Autodesk Inventor part; units mm, degrees
ref_plane "YZ Plane" through (0, 0, 0) normal (1, 0, 0) x (0, 1, 0)
ref_plane "XZ Plane" through (0, 0, 0) normal (0, 1, 0) x (-1, 0, 0)
ref_plane "XY Plane" through (0, 0, 0) normal (0, 0, 1) x (1, 0, 0)
sketch "Sketch1" plane through (0, 0, 0) normal (0, 0, 1) x (1, 0, 0)
  line L0 (229.6952, -414.7737) -> (228.902, -414.7737)
  line L1 (204.202, -567.6898) -> (204.202, -542.0358)
  line L2 (204.202, -542.0358) -> (229.856, -542.0358)
  line L3 (204.202, -567.6898) -> (-74.944, -567.6898)
  line L4 (-74.944, -567.6898) -> (-74.944, -265.633)
  line L5 (229.856, -542.0358) -> (229.856, -8.8898)
  line L6 (229.856, -8.8898) -> (188.7123, -8.8898)
  circle A0 centre (20.5783, -308.8638) radius 3.5687
  circle A1 centre (20.574, -385.0638) radius 3.5687
  circle A2 centre (20.574, -461.2638) radius 3.5687
  circle A3 centre (20.574, -537.4638) radius 3.5687
  circle A4 centre (217.156, -529.3358) radius 3.5687
  circle A5 centre (209.282, -461.2638) radius 3.5687
  circle A6 centre (209.282, -385.0638) radius 3.5687
  circle A7 centre (209.282, -308.8638) radius 3.5687
  circle A8 centre (209.282, -232.6638) radius 3.5687
  circle A9 centre (209.2863, -156.4638) radius 3.5687
  circle A10 centre (209.282, -80.2638) radius 3.5687
  circle A11 centre (209.282, -29.4638) radius 3.5687
  line L7 (229.856, -8.8898) -> (-74.944, -8.8898)
  line L8 (-74.944, -8.8898) -> (-74.944, -567.6898)
  line L9 (191.756, -567.6898) -> (37.6288, -567.6898)
  line L10 (37.6288, -567.6898) -> (37.6288, -435.6098)
  line L11 (37.6288, -435.6098) -> (191.756, -435.6098)
  line L12 (191.756, -435.6098) -> (191.756, -567.6898)
  circle A12 centre (1.256, -76.1998) radius 189.4332 construction
  circle A13 centre (1.256, -76.1998) radius 14.2875
  point P0 (0, 0)
  dimension "d0" = 25.654
  dimension "d3" = 558.8
  dimension "d5" = 76.2
  dimension "d6" = 20.5697
  dimension "d7" = 20.574
  dimension "d9" = 76.2
  dimension "d10" = 76.2
  dimension "d11" = 76.2
  dimension "d12" = 76.2
  dimension "d13" = 25.654
  dimension "d14" = 12.7
  dimension "d15" = 76.2
  dimension "d16" = 76.2
  dimension "d17" = 76.2
  dimension "d18" = 43.2308
  dimension "d23" = 7.1374
  dimension "d24" = 7.1374
  dimension "d25" = 7.1374
  dimension "d26" = 7.1374
  dimension "d27" = 7.1374
  dimension "d28" = 7.1374
  dimension "d29" = 7.1374
  dimension "d30" = 7.1374
  dimension "d31" = 7.1374
  dimension "d32" = 7.1374
  dimension "d33" = 7.1374
  dimension "d34" = 7.1374
  dimension "d35" = 304.8
  dimension "d36" = 12.7
  dimension "d37" = 106.426
  dimension "d38" = 188.7037
  dimension "d39" = 188.708
  dimension "d40" = 188.708
  dimension "d41" = 188.708
  dimension "d42" = 20.574
  dimension "d43" = 20.574
  dimension "d44" = 20.574
  dimension "d45" = 30.226
  dimension "d46" = 20.574
  dimension "d47" = 12.446
  dimension "d48" = 154.1272
  dimension "d49" = 132.08
  dimension "d50" = 378.8664
  dimension "d51" = 76.2
  dimension "d56" = 491.49
  dimension "d57" = 28.575
  dimension "d61" = 50.8
extrude "Extrusion1" add sketch "Sketch1" along normal blind 3.175 contours L3 L12 L11 L10 L4 L8 L7 L6 L5 L2 L1
sketch "Sketch2" plane through (0, 0, 3.175) normal (0, 0, 1) x (1, 0, 0)
  point P0 (0, 0)
properties part number "GearboxPlateRev3"
Here's how the part is built. I have some questions about the finished solid (model axes, mm). Coordinates: 2 decimals unless noted, no trailing zeros. Loops run counter-clockwise (first coordinate to the right, second up) from the corner with the lowest first, then second, coordinate; pieces in that order, holes last.
1. Imagine slicing it at C-C, the plane z = 1.45. Count the separate pieces of the cut face and the enclosed holes in it, and give its area (3 significant figures).
2. Imagine slicing it at B-B, the plane x = -1. Please give me the cut outline in (y, z) (3 decimals), and give its area (3 significant figures).
3. Imagine slicing it at A-A, the plane y = -501. Please give me the cut outline in (x, z) (3 decimals), and give its area (3 significant figures).
4. I need wall thicknesses on L1, parallel to X at y = -308, z = 2.15; L2, parallel to X at y = -76, z = 1.5; L3, parallel to Y at x = 187.5, z = 2.4. Which ranges of each line are inside material? Lowest first, please.
5. Imagine slicing it at D-D, the plane x = 95. Please give me the cut outline in (y, z) (3 decimals), and give its area (3 significant figures).
6. For P1, Ø11.5, axis at x = 20.57, y = -537.46, coming from the -Z side; P2, Ø1, axis at x = 122, z = 1, coming from the -Y side, each with a flat end and sliding along its axis, tell me the tip position at first contact or that it passes through.
Taken from the geometry:
1. separate pieces: 1
1. enclosed holes: 13
1. area: 148,000 mm2
2. outline: (-567.69, 0) - (-90.308, 0) - (-90.308, 3.175) - (-567.69, 3.175) - close; (-62.092, 0) - (-8.89, 0) - (-8.89, 3.175) - (-62.092, 3.175) - close
2. area: 1,680 mm2
3. outline: (-74.944, 0) - (37.629, 0) - (37.629, 3.175) - (-74.944, 3.175) - close; (191.756, 0) - (229.856, 0) - (229.856, 3.175) - (191.756, 3.175) - close
3. area: 478 mm2
4. L1: x = -74.94 to 17.12, 24.04 to 205.82, 212.74 to 229.86
4. L2: x = -74.94 to -13.03, 15.54 to 229.86
4. L3: y = -435.61 to -8.89
5. outline: (-435.61, 0) - (-8.89, 0) - (-8.89, 3.175) - (-435.61, 3.175) - close
5. area: 1,350 mm2
6. P1: stops at z = 0
6. P2: stops at y = -435.61
